The listing builds one solid part. Answer for the finished solid, in the listing's coordinates (mm). Coordinates: 2 decimals unless noted, no trailing zeros. Loops run counter-clockwise (first coordinate to the right, second up) from the corner with the lowest first, then second, coordinate; pieces in that order, holes last. Notation, with made-up numbers: M -31,87 L 19,87 A25 cw 19,125 Z; hole C 68.25,-19 d6. An arc over 180 degrees is marked long. Answer as a JSON object with one key per item and string values. Group by question number.
1. Given pin 1 (1.3 mm diameter, centred on y = 21.5, z = 4.5, fed in from -X), flat-ended and moving along its own axis, determine where the tip first touches the part or whether it passes through.
2. Determine the mould class of faces 1 (the face through (72, 69.325, 5)), 2 (the face through (0, 45, 5)), 3 (the face through (95.6, 45, 5)), 4 (the face through (75.575, 64, 5)) for opening direction X: released by +X, released by -X, zero draft, split by the parting line, or undercut.
3. A cutting plane is placed at B-B on x = 36.5. Give the vertices of the cut face in (y, z) (3 decimals), and give its area (4 significant figures).
4. Straight lines are drawn through the part: L1, parallel to Y at x = 62, z = 5.5 (3 decimals); L2, parallel to X at y = 29, z = 7.75; L3, parallel to X at y = 57.5, z = 0.75 (3 decimals). For each, find the intervals that lie inside material, in ascending order.
5. A cutting plane is placed at A-A on y = 25. Give the vertices of the cut face in (x, z).
6. A cutting plane is placed at C-C on z = 4. State how many separate pieces and enclosed holes the cut face has, and give its area (3 significant figures).
from build123d import *

# Parameters (mm, degrees)
F0_W     = 95.6
F0_H     = 91.7
F1_DEPTH = 10


with BuildPart() as f1:
    # F0 (on Top) → F1 (new body)
    with BuildSketch(Plane.XY):
        with Locations((47.8, 45.85)):
            Rectangle(F0_W, F0_H)
        with BuildLine():
            ThreePointArc((29.025, 33.5), (29.166421, 33.558579), (29.225, 33.7))
            Line((29.225, 33.7), (29.225, 34.925))
            ThreePointArc((29.225, 34.925), (30.15, 35.85), (31.075, 34.925))
            Line((31.075, 34.925), (31.075, 33.7))
            ThreePointArc((31.075, 33.7), (31.133579, 33.558579), (31.275, 33.5))
            Line((31.275, 33.5), (39.817157, 33.5))
            ThreePointArc((39.817157, 33.5), (39.874892, 33.51835), (39.911438, 33.566667))
            ThreePointArc((39.911438, 33.566667), (40.13382, 33.69712), (40.3, 33.5))
            Line((40.3, 33.5), (40.3, 22.35))
            ThreePointArc((40.3, 22.35), (40.13382, 22.15288), (39.911438, 22.283333))
            ThreePointArc((39.911438, 22.283333), (39.874892, 22.33165), (39.817157, 22.35))
            Line((39.817157, 22.35), (31.275, 22.35))
            ThreePointArc((31.275, 22.35), (31.133579, 22.291421), (31.075, 22.15))
            Line((31.075, 22.15), (31.075, 20.925))
            ThreePointArc((31.075, 20.925), (30.15, 20), (29.225, 20.925))
            Line((29.225, 20.925), (29.225, 22.15))
            ThreePointArc((29.225, 22.15), (29.166421, 22.291421), (29.025, 22.35))
            Line((29.025, 22.35), (20.482843, 22.35))
            ThreePointArc((20.482843, 22.35), (20.425108, 22.33165), (20.388562, 22.283333))
            ThreePointArc((20.388562, 22.283333), (20.16618, 22.15288), (20, 22.35))
            Line((20, 22.35), (20, 33.5))
            ThreePointArc((20, 33.5), (20.16618, 33.69712), (20.388562, 33.566667))
            ThreePointArc((20.388562, 33.566667), (20.425108, 33.51835), (20.482843, 33.5))
            Line((20.482843, 33.5), (29.025, 33.5))
        make_face(mode=Mode.SUBTRACT)
        with BuildLine():
            ThreePointArc((66.825, 33.5), (66.966421, 33.558579), (67.025, 33.7))
            Line((67.025, 33.7), (67.025, 34.925))
            ThreePointArc((67.025, 34.925), (67.95, 35.85), (68.875, 34.925))
            Line((68.875, 34.925), (68.875, 33.7))
            ThreePointArc((68.875, 33.7), (68.933579, 33.558579), (69.075, 33.5))
            Line((69.075, 33.5), (75.117157, 33.5))
            ThreePointArc((75.117157, 33.5), (75.174892, 33.51835), (75.211438, 33.566667))
            ThreePointArc((75.211438, 33.566667), (75.43382, 33.69712), (75.6, 33.5))
            Line((75.6, 33.5), (75.6, 22.35))
            ThreePointArc((75.6, 22.35), (75.43382, 22.15288), (75.211438, 22.283333))
            ThreePointArc((75.211438, 22.283333), (75.174892, 22.33165), (75.117157, 22.35))
            Line((75.117157, 22.35), (69.075, 22.35))
            ThreePointArc((69.075, 22.35), (68.933579, 22.291421), (68.875, 22.15))
            Line((68.875, 22.15), (68.875, 20.925))
            ThreePointArc((68.875, 20.925), (67.95, 20), (67.025, 20.925))
            Line((67.025, 20.925), (67.025, 22.15))
            ThreePointArc((67.025, 22.15), (66.966421, 22.291421), (66.825, 22.35))
            Line((66.825, 22.35), (60.782843, 22.35))
            ThreePointArc((60.782843, 22.35), (60.725108, 22.33165), (60.688562, 22.283333))
            ThreePointArc((60.688562, 22.283333), (60.46618, 22.15288), (60.3, 22.35))
            Line((60.3, 22.35), (60.3, 33.5))
            ThreePointArc((60.3, 33.5), (60.46618, 33.69712), (60.688562, 33.566667))
            ThreePointArc((60.688562, 33.566667), (60.725108, 33.51835), (60.782843, 33.5))
            Line((60.782843, 33.5), (66.825, 33.5))
        make_face(mode=Mode.SUBTRACT)
        with BuildLine():
            ThreePointArc((29.025, 69.325), (29.166421, 69.383579), (29.225, 69.525))
            Line((29.225, 69.525), (29.225, 70.775))
            ThreePointArc((29.225, 70.775), (30.15, 71.7), (31.075, 70.775))
            Line((31.075, 70.775), (31.075, 69.525))
            ThreePointArc((31.075, 69.525), (31.133579, 69.383579), (31.275, 69.325))
            Line((31.275, 69.325), (39.792157, 69.325))
            ThreePointArc((39.792157, 69.325), (39.849892, 69.34335), (39.886438, 69.391667))
            ThreePointArc((39.886438, 69.391667), (40.10882, 69.52212), (40.275, 69.325))
            Line((40.275, 69.325), (40.275, 58.225))
            ThreePointArc((40.275, 58.225), (40.10882, 58.02788), (39.886438, 58.158333))
            ThreePointArc((39.886438, 58.158333), (39.849892, 58.20665), (39.792157, 58.225))
            Line((39.792157, 58.225), (31.275, 58.225))
            ThreePointArc((31.275, 58.225), (31.133579, 58.166421), (31.075, 58.025))
            Line((31.075, 58.025), (31.075, 56.775))
            ThreePointArc((31.075, 56.775), (30.15, 55.85), (29.225, 56.775))
            Line((29.225, 56.775), (29.225, 58.025))
            ThreePointArc((29.225, 58.025), (29.166421, 58.166421), (29.025, 58.225))
            Line((29.025, 58.225), (20.507843, 58.225))
            ThreePointArc((20.507843, 58.225), (20.450108, 58.20665), (20.413562, 58.158333))
            ThreePointArc((20.413562, 58.158333), (20.19118, 58.02788), (20.025, 58.225))
            Line((20.025, 58.225), (20.025, 69.325))
            ThreePointArc((20.025, 69.325), (20.19118, 69.52212), (20.413562, 69.391667))
            ThreePointArc((20.413562, 69.391667), (20.450108, 69.34335), (20.507843, 69.325))
            Line((20.507843, 69.325), (29.025, 69.325))
        make_face(mode=Mode.SUBTRACT)
        with BuildLine():
            ThreePointArc((66.825, 69.325), (66.966421, 69.383579), (67.025, 69.525))
            Line((67.025, 69.525), (67.025, 70.775))
            ThreePointArc((67.025, 70.775), (67.95, 71.7), (68.875, 70.775))
            Line((68.875, 70.775), (68.875, 69.525))
            ThreePointArc((68.875, 69.525), (68.933579, 69.383579), (69.075, 69.325))
            Line((69.075, 69.325), (75.092157, 69.325))
            ThreePointArc((75.092157, 69.325), (75.149892, 69.34335), (75.186438, 69.391667))
            ThreePointArc((75.186438, 69.391667), (75.40882, 69.52212), (75.575, 69.325))
            Line((75.575, 69.325), (75.575, 58.225))
            ThreePointArc((75.575, 58.225), (75.40882, 58.02788), (75.186438, 58.158333))
            ThreePointArc((75.186438, 58.158333), (75.149892, 58.20665), (75.092157, 58.225))
            Line((75.092157, 58.225), (69.075, 58.225))
            ThreePointArc((69.075, 58.225), (68.933579, 58.166421), (68.875, 58.025))
            Line((68.875, 58.025), (68.875, 56.775))
            ThreePointArc((68.875, 56.775), (67.95, 55.85), (67.025, 56.775))
            Line((67.025, 56.775), (67.025, 58.025))
            ThreePointArc((67.025, 58.025), (66.966421, 58.166421), (66.825, 58.225))
            Line((66.825, 58.225), (60.807843, 58.225))
            ThreePointArc((60.807843, 58.225), (60.750108, 58.20665), (60.713562, 58.158333))
            ThreePointArc((60.713562, 58.158333), (60.49118, 58.02788), (60.325, 58.225))
            Line((60.325, 58.225), (60.325, 69.325))
            ThreePointArc((60.325, 69.325), (60.49118, 69.52212), (60.713562, 69.391667))
            ThreePointArc((60.713562, 69.391667), (60.750108, 69.34335), (60.807843, 69.325))
            Line((60.807843, 69.325), (66.825, 69.325))
        make_face(mode=Mode.SUBTRACT)
    extrude(amount=F1_DEPTH)


solid = f1.part
From the geometry:
{
 "1": {"pin 1": "stops at x = 0"},
 "2": {"face 1": "undercut", "face 2": "released by -X", "face 3": "released by +X", "face 4": "undercut"},
 "3": {"outline": "M 0,0 L 22.35,0 L 22.35,10 L 0,10 Z; M 33.5,0 L 58.225,0 L 58.225,10 L 33.5,10 Z; M 69.325,0 L 91.7,0 L 91.7,10 L 69.325,10 Z", "area": "694.5 mm²"},
 "4": {"L1": "y = 0 to 22.35, 33.5 to 58.225, 69.325 to 91.7", "L2": "x = 0 to 20, 40.3 to 60.3, 75.6 to 95.6", "L3": "x = 0 to 29.225, 31.075 to 67.025, 68.875 to 95.6"},
 "5": {"outline": "M 0,0 L 20,0 L 20,10 L 0,10 Z; M 40.3,0 L 60.3,0 L 60.3,10 L 40.3,10 Z; M 75.6,0 L 95.6,0 L 95.6,10 L 75.6,10 Z"},
 "6": {"separate pieces": "1", "enclosed holes": "4", "area": "7,940 mm²"}
}
